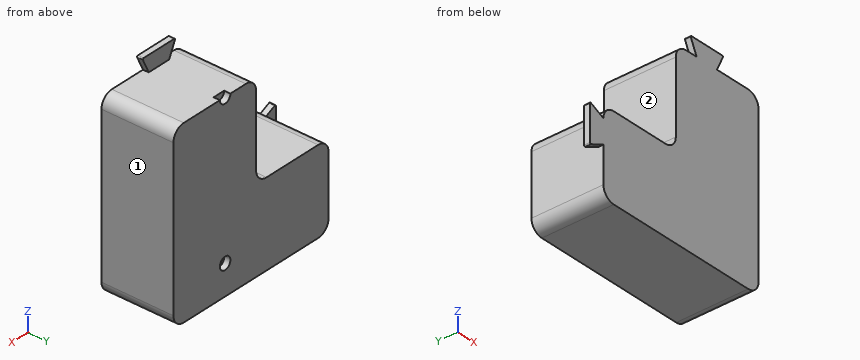
Autodesk Inventor part; units mm, degrees
ref_plane "YZ Plane" through (0, 0, 0) normal (1, 0, 0) x (0, 1, 0)
ref_plane "XZ Plane" through (0, 0, 0) normal (0, 1, 0) x (-1, 0, 0)
ref_plane "XY Plane" through (0, 0, 0) normal (0, 0, 1) x (1, 0, 0)
sketch "Sketch1" plane through (0, 0, 0) normal (0, 1, 0) x (-1, 0, 0)
  line L0 (0, 0) -> (200, 0)
  line L1 (200, 0) -> (200, 200)
  line L2 (200, 200) -> (0, 200)
  line L3 (0, 200) -> (0, 0)
  line L4 (110, 199.8) -> (110, 213.2303) construction
  line L5 (100, 213.1946) -> (114.7696, 213.1946)
  arc A0 (115.4946, 212.0565) -> (114.7696, 213.1946) centre (114.7696, 212.3946) ccw
  line L6 (115.4946, 212.0565) -> (109.8726, 200)
  line L7 (109.8726, 200) -> (90.1274, 200)
  line L8 (90.1274, 200) -> (84.5054, 212.0565)
  arc A1 (85.2304, 213.1946) -> (84.5054, 212.0565) centre (85.2304, 212.3946) ccw
  line L9 (85.2304, 213.1946) -> (100, 213.1946)
  line L10 (200, 89.8726) -> (200, 110.1274)
  line L11 (200, 90.1274) -> (200, 109.8726)
  line L12 (200, 109.8726) -> (212.0565, 115.4946)
  arc A2 (213.1946, 114.7696) -> (212.0565, 115.4946) centre (212.3946, 114.7696) ccw
  line L13 (213.1946, 114.7696) -> (213.1946, 100)
  line L14 (199.8, 90) -> (213.2303, 90) construction
  line L15 (212.0565, 84.5054) -> (200, 90.1274)
  line L16 (213.1946, 100) -> (213.1946, 85.2304)
  arc A3 (212.0565, 84.5054) -> (213.1946, 85.2304) centre (212.3946, 85.2304) ccw
  point P0 (0, 100)
  point P1 (0, 100)
  point P2 (0, 100)
  point P3 (0, 100)
  point P4 (100, 200)
  point P5 (100, 200)
  point P6 (100, 200)
  point P7 (100, 200)
  point P8 (100, 200)
  point P9 (100, 200)
  point P10 (200, 100)
  point P11 (200, 100)
  point P12 (200, 100)
  point P13 (200, 100)
  point P14 (200, 100)
  point P15 (200, 100)
  point P16 (200, 100)
  point P17 (200, 100)
  point P18 (200, 100)
  point P19 (200, 100)
  dimension "d0" = 200
  dimension "d1" = 200
extrude "Extrusion1" add sketch "Sketch1" along normal blind 60 contours L3 L2 L1 L0
extrude "Extrusion3" add sketch "Sketch1" along normal blind 4.8 contours L8 A1 L9 L5 A0 L6 L2 | L1 L12 A2 L13 L16 A3 L15
sketch "Sketch2" plane through (0, 60, 0) normal (0, 1, 0) x (1, 0, 0)
  line L0 (0, 0) -> (-200, 0)
  circle A0 centre (-100, -75) radius 5.1
  circle A1 centre (-100, -200) radius 5.1
  dimension "d11" = 10.2
  dimension "d12" = 10.2
extrude "Extrusion4" cut sketch "Sketch2" against normal blind 5.2
sketch "Sketch3" plane through (0, 60, 0) normal (0, 1, 0) x (1, 0, 0)
  line L0 (0, -200) -> (0, 0)
  line L1 (-94.9, -200) -> (0, -200)
  line L2 (0, 0) -> (-70, 0)
  line L3 (-70, 0) -> (-70, -200)
  line L4 (-70, -200) -> (0, -200)
  line L5 (0, -200) -> (0, 0)
  line L6 (-200, 0) -> (-200, -200)
  line L7 (-200, 0) -> (0, 0)
  line L8 (0, 0) -> (0, -50)
  line L9 (0, -50) -> (-200, -50)
  line L10 (-200, -50) -> (-200, 0)
  line L11 (-200, -200) -> (-130, -200)
  line L12 (-130, -200) -> (-130, -120)
  line L13 (-130, -120) -> (-200, -120)
  line L14 (-200, -120) -> (-200, -200)
  point P0 (-70, -50)
  dimension "d17" = 70
  dimension "d18" = 50
  dimension "d19" = 70
  dimension "d20" = 80
extrude "Extrusion6" cut sketch "Sketch3" against normal blind 60
sketch "Sketch4" plane through (-70, 60, 200) normal (1, 0, 0) x (0, 0, -1)
  line L0 (150, -60) -> (109.8726, -60)
  line L1 (0, 0) -> (150, 0)
  line L2 (150, 0) -> (150, -60)
  line L3 (150, -60) -> (0, -60)
  line L4 (0, -60) -> (0, 0)
  point P0 (200, -60)
extrude "Extrusion7" add sketch "Sketch4" along normal blind 20
fillet "Fillet2" radius 10 6 edges at (-50, 30, 50) (-200, 30, 50) (-50, 30, 200) (-130, 30, 200) (-130, 30, 120) (-200, 30, 120)
properties part number "Area øv1"
The listing builds one solid part. Answer for the finished solid, in the listing's coordinates (mm). Face numbers are marked on the shaded views. A direction names the side the tool comes from. Give positions to 0.01 mm unless a question says otherwise; leave off trailing zeros. Order: outer loops, then holes, each group sorted by start corner. A loop starts at its lowest first (then second) coordinate and runs counter-clockwise, first axis right, second up. Notation, with made-up numbers: (-13.75, 18.25) -> (5.25, 18.25) arc R18 cw to (5.25, 28.25) -> close; hole circle Ø7 at (-5, 6). An arc over 180 degrees is marked (long way). Write each question's results on one line, items separated by ' | '.
Q1. The part is cut by section C-C, the plane y = 23.5. Give the vertices of the cut face in (x, z).
Checked values:
outline: (-200, 60) arc R10 ccw to (-190, 50) -> (-60, 50) arc R10 ccw to (-50, 60) -> (-50, 190) arc R10 ccw to (-60, 200) -> (-120, 200) arc R10 ccw to (-130, 190) -> (-130, 130) arc R10 cw to (-140, 120) -> (-190, 120) arc R10 ccw to (-200, 110) -> close
Q2. Straight lines are drawn through the part: probe 1 along Z at (x, y) = (-100, 56.9); probe 2 along X at (y, z) = (57, 75); probe 3 along X at (y, z) = (12, 70.5). For each, find the intervals that lie inside material, in ascending order. Write a range as from..to.
Checked values:
probe 1: z = 50..69.9, 80.1..194.9 | probe 2: x = -200..-105.1, -94.9..-50 | probe 3: x = -200..-50
Q3. Each of these flat-tipped pins is pushed along its axis until it touches: P1, Ø15, axis at y = 20, z = 89.5, coming from the -X side; P2, Ø10.5, axis at x = -107, z = 209, coming from the +Y side; P3, Ø18, axis at y = 41, z = 165, coming from the -X side. Where does it stop, or does it pass through?
Checked values:
P1: stops at x = -200 | P2: stops at y = 4.8 | P3: stops at x = -130
Q4. The part is cut by section D-D, the plane x = -171. Give the vertices of the cut face in (y, z), and give its area (3 significant figures).
Checked values:
outline: (0, 50) -> (60, 50) -> (60, 120) -> (0, 120) -> close | area: 4,200 mm^2
Q5. Which of the six approach directions +Z, -Z, +X, -X, +Y, -Y give full straight-line access (tool end or side, diameter ignored) to the marked faces 1 and 2?
Checked values:
face 1: +Z, -Z, +X, +Y, -Y | face 2: +Z, -X, +Y, -Y
Q6. The part is cut by section A-A, the plane x = -100. Give the vertices of the cut face in (y, z), and give its area (3 significant figures).
Checked values:
outline: (0, 50) -> (60, 50) -> (60, 69.9) -> (54.8, 69.9) -> (54.8, 80.1) -> (60, 80.1) -> (60, 194.9) -> (54.8, 194.9) -> (54.8, 200) -> (4.8, 200) -> (4.8, 213.19) -> (0, 213.19) -> close | area: 8,980 mm^2
Q7. The part is cut by section B-B, the plane z = 75. Give the vertices of the cut face in (x, y), and give its area (3 significant figures).
Checked values:
outline: (-200, 0) -> (-50, 0) -> (-50, 60) -> (-94.9, 60) -> (-94.9, 54.8) -> (-105.1, 54.8) -> (-105.1, 60) -> (-200, 60) -> close | area: 8,950 mm^2
